Check sheet for the drawn part. Datum: minimum x, y, z corner. Units: mm. A direction names the side the tool comes from. Coordinates: 2 decimals unless noted, no trailing zeros. Order: outer loops, then holes, each group sorted by start corner. A loop starts at its lowest first (then second) coordinate and runs counter-clockwise, first axis right, second up.
Q1. Cross-section at D-D, the plane x = 33. Record the boundary of the cut face in (y, z), and give its area (3 significant figures).
Q2. Cross-section at B-B, the plane y = 2.5. Record the boundary of the cut face in (x, z).
Q3. Depth check by flat-ended pin: P1, Ø4, axis at x = 30.91, z = 12, coming from the +Y side; P2, Ø2.5, axis at x = 19, y = 7, coming from the -Z side; P3, Ø0.6, axis at y = 10.5, z = 43, coming from the -X side; P4, Ø1.8, axis at x = 10.91, z = 32, coming from the -Y side. Enter the tip coordinate at first touch or a pass-through.
Q4. Draft check along Z on the marked faces 1, 2 and 3. Enter one of: pulls with the +Z half, pulls with the -Z half, needs draft (parallel to the pull), parting line crosses it, or undercut.
Q5. Set-up check for the marked faces 4 and 5: record each of +Z, -Z, +X, -X, +Y, -Y from which the full face is reachable in a straight line by a thin tool's end or side.
Q6. Cross-section at A-A, the plane x = 27. Record the boundary of the cut face in (y, z).
Q7. Cross-section at C-C, the plane z = 12. Record the boundary of the cut face in (x, y).
Q8. Thickness scan on line 1 (X direction, y = 7, z = 0.65); line 2 (Z direction, x = 24.5, y = 5); line 3 (Y direction, x = 19, z = 1.45). Record the ranges inside material, lowest first.
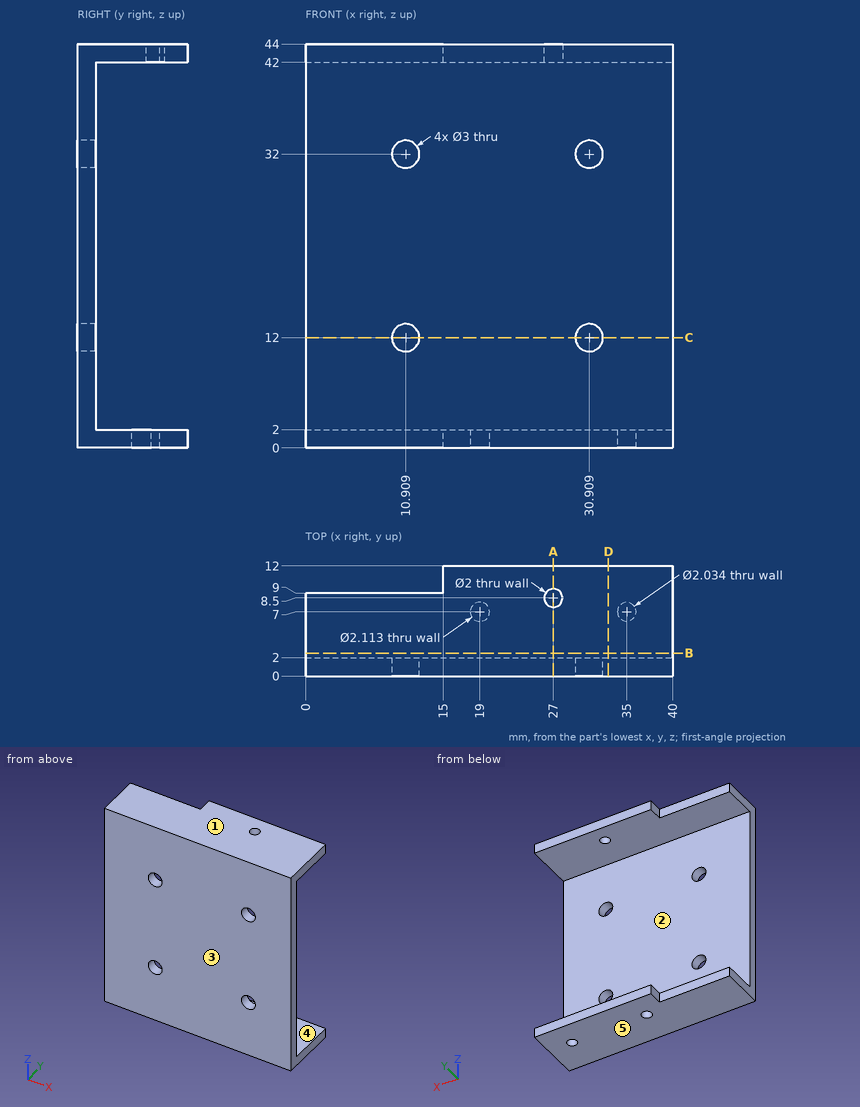
Check values:
1. outline: (0, 0) - (12, 0) - (12, 2) - (2, 2) - (2, 42) - (12, 42) - (12, 44) - (0, 44) - close
1. area: 128 mm2
2. outline: (0, 0) - (40, 0) - (40, 2) - (0, 2) - close; (0, 42) - (40, 42) - (40, 44) - (0, 44) - close
3. P1: stops at y = 2
3. P2: stops at z = 0
3. P3: stops at x = 15
3. P4: passes through
4. face 1: pulls with the +Z half
4. face 2: undercut
4. face 3: needs draft
5. face 4: +X, -X, +Y
5. face 5: -Z, +X, -X, +Y, -Y
6. outline: (0, 0) - (12, 0) - (12, 2) - (2, 2) - (2, 42) - (7.5, 42) - (7.5, 44) - (0, 44) - close; (9.5, 42) - (12, 42) - (12, 44) - (9.5, 44) - close
7. outline: (0, 0) - (9.41, 0) - (9.41, 2) - (0, 2) - close; (12.41, 0) - (29.41, 0) - (29.41, 2) - (12.41, 2) - close; (32.41, 0) - (40, 0) - (40, 2) - (32.41, 2) - close
8. line 1: x = 0 to 17.94, 20.06 to 33.98, 36.02 to 40
8. line 2: z = 0 to 2, 42 to 44
8. line 3: y = 0 to 5.94, 8.06 to 12
